CAD build for the part. Positions are in the model's coordinates, mm. A direction names the side the tool comes from. Give positions to 0.01 mm unless a question says otherwise; leave off trailing zeros. Loops run counter-clockwise (first coordinate to the right, second up) from the corner with the lowest first, then second, coordinate; pieces in that order, holes last.
```python
from build123d import *

# Parameters (mm, degrees)
SKETCH2_W                      = 230
SKETCH2_H                      = 283.251
BOSS_EXTRUDE1_DEPTH            = 10
SKETCH3_W                      = 10
SKETCH3_H                      = 283.251
BOSS_EXTRUDE2_DEPTH            = 170
M6_CLEARANCE_HOLE1_D           = 7
CUT_EXTRUDE1_DEPTH             = 327.431895271
CUT_EXTRUDE1_DEPTH_BACK        = 327.431895271
SKETCH7_R                      = 3.81
SKETCH7_R_2                    = 1.89865
SKETCH8_W                      = 6.35
SKETCH8_H                      = 38.1
CUT_EXTRUDE2_DEPTH             = 36.025
CUT_EXTRUDE3_DEPTH             = 6.35
CUT_EXTRUDE4_REACH             = 331.125
SKETCH11_R                     = 3.81
F_6_CLEARANCE_HOLE1_D          = 3.7973
F_6_CLEARANCE_HOLE1_DEPTH      = 3.65
CIRPATTERN1_COUNT              = 2
ENL_V_MAT_EXTRU_1_REACH        = 249.554
ESQUISSE1_R                    = 3.175
CBORE_FOR_M5_SHCS1_D           = 5.5
CBORE_FOR_M5_SHCS1_CBORE_D     = 10
CBORE_FOR_M5_SHCS1_CBORE_DEPTH = 5
CUT_EXTRUDE5_DEPTH             = 248.553594703
CUT_EXTRUDE5_DEPTH_BACK        = 248.553594703
SKETCH15_W                     = 58.825
SKETCH15_H                     = 59.331356017
CUT_EXTRUDE7_DEPTH             = 248.553594703
CUT_EXTRUDE7_DEPTH_BACK        = 248.553594703
SKETCH20_W                     = 0.765
SKETCH20_H                     = 59.331356017
FILLET2_R                      = 4
FILLET3_R                      = 144
FILLET4_R                      = 4
CUT_EXTRUDE8_REACH             = 335.853
CUT_EXTRUDE9_REACH             = 335.853
FILLET5_R                      = 8
FILLET6_R                      = 8
FILLET7_R                      = 10


with BuildPart() as part:
    # Sketch2 → Boss-Extrude1 (new body)
    with BuildSketch(Plane(origin=(0, 0, 0), x_dir=(1, 0, 0), z_dir=(0, 1, 0))):
        Rectangle(SKETCH2_W, SKETCH2_H)
    extrude(amount=BOSS_EXTRUDE1_DEPTH)

    # Sketch3 → Boss-Extrude2 (add)
    with BuildSketch(Plane(origin=(0, 0, 0), x_dir=(1, 0, 0), z_dir=(0, 1, 0))):
        with Locations((-120, 0)):
            Rectangle(SKETCH3_W, SKETCH3_H)
        with Locations((120, 0)):
            Rectangle(SKETCH3_W, SKETCH3_H)
    extrude(amount=BOSS_EXTRUDE2_DEPTH)

    # M6 Clearance Hole1 (through all)
    with Locations(Plane(origin=(0, 10, 0), x_dir=(1, 0, 0), z_dir=(0, 1, 0))):
        with Locations((-25, 25), (25, 25), (25, -25), (-25, -25)):
            Hole(M6_CLEARANCE_HOLE1_D / 2)

    # Sketch7 → Cut-Extrude1 (cut, two sides: drawn at the far end of the back side and taken through both)
    with BuildSketch(Plane.ZY.offset(-115).offset(-CUT_EXTRUDE1_DEPTH_BACK)):
        with Locations((0, 153.49)):
            Circle(SKETCH7_R)
        with Locations((0, 163.269)):
            Circle(SKETCH7_R_2)
        with Locations((6.914797213, 160.404797213)):
            Circle(SKETCH7_R_2)
        with Locations((9.779, 153.49)):
            Circle(SKETCH7_R_2)
        with Locations((6.914797213, 146.575202787)):
            Circle(SKETCH7_R_2)
        with Locations((0, 143.711)):
            Circle(SKETCH7_R_2)
        with Locations((-6.914797213, 146.575202787)):
            Circle(SKETCH7_R_2)
        with Locations((-9.779, 153.49)):
            Circle(SKETCH7_R_2)
        with Locations((-6.914797213, 160.404797213)):
            Circle(SKETCH7_R_2)
    extrude(amount=CUT_EXTRUDE1_DEPTH + CUT_EXTRUDE1_DEPTH_BACK, mode=Mode.SUBTRACT)

    # Sketch8 → Cut-Extrude2 (cut)
    with BuildSketch(Plane(origin=(0, 170, 0), x_dir=(1, 0, 0), z_dir=(0, 1, 0))):
        with Locations((121.825, 0)):
            Rectangle(SKETCH8_W, SKETCH8_H)
        with Locations((-121.825, 0)):
            Rectangle(SKETCH8_W, SKETCH8_H)
    extrude(amount=-CUT_EXTRUDE2_DEPTH, mode=Mode.SUBTRACT)

    # Sketch9 → Cut-Extrude3 (cut)
    with BuildSketch(Plane(origin=(125, 0, 0), x_dir=(0, 0, -1), z_dir=(1, 0, 0))):
        Polygon((72.294143983, 74.514), (72.294143983, 35.986), (34.274143983, 35.986), (34.274143983, 74.514), (34.274143983, 170), (72.294143983, 170), align=None)
    cut_extrude3 = extrude(amount=-CUT_EXTRUDE3_DEPTH, mode=Mode.SUBTRACT)

    # Sketch11 → Cut-Extrude4 (cut, up to next)
    with BuildSketch(Plane(origin=(118.65, 0, 0), x_dir=(0, 0, -1), z_dir=(1, 0, 0)), mode=Mode.PRIVATE) as cut_extrude4_sk1:
        with Locations((53.284143983, 55.25)):
            Circle(SKETCH11_R)
    cut_extrude4_tool1 = extrude(cut_extrude4_sk1.sketch, amount=-CUT_EXTRUDE4_REACH, mode=Mode.PRIVATE) & part.part
    cut_extrude4 = cut_extrude4_tool1.solids().sort_by_distance((118.65, 55.25, -53.284144))[0]
    add(cut_extrude4, mode=Mode.SUBTRACT)

    # #6 Clearance Hole1
    with Locations(Plane(origin=(118.65, 0, 0), x_dir=(0, 0, -1), z_dir=(1, 0, 0))):
        with Locations((53.284143983, 65.029), (43.505143983, 55.25), (63.063143983, 55.25), (53.284143983, 45.471)):
            f_6_clearance_hole1 = Hole(F_6_CLEARANCE_HOLE1_D / 2, depth=F_6_CLEARANCE_HOLE1_DEPTH)

    # CirPattern1: Cut-Extrude3, Cut-Extrude4, #6 Clearance Hole1 ×2 about axis
    cirpattern1_axis = Axis((0, 0, 0), (0, 1, 0))
    add([cut_extrude3.rotate(cirpattern1_axis, i * 360 / CIRPATTERN1_COUNT) for i in range(1, CIRPATTERN1_COUNT)], mode=Mode.SUBTRACT)
    add([cut_extrude4.rotate(cirpattern1_axis, i * 360 / CIRPATTERN1_COUNT) for i in range(1, CIRPATTERN1_COUNT)], mode=Mode.SUBTRACT)
    add([f_6_clearance_hole1.rotate(cirpattern1_axis, i * 360 / CIRPATTERN1_COUNT) for i in range(1, CIRPATTERN1_COUNT)], mode=Mode.SUBTRACT)

    # Esquisse1 → Enlèv. mat.-Extru.1 (cut, up to next)
    with BuildSketch(Plane(origin=(0, 10, 0), x_dir=(1, 0, 0), z_dir=(0, 1, 0)), mode=Mode.PRIVATE) as enl_v_mat_extru_1_sk1:
        with Locations(Location((53, 82.268595163, 0), (0, 0, 270))):
            Circle(ESQUISSE1_R)
    enl_v_mat_extru_1_tool1 = extrude(enl_v_mat_extru_1_sk1.sketch, amount=-ENL_V_MAT_EXTRU_1_REACH, mode=Mode.PRIVATE) & part.part
    # Esquisse1 → Enlèv. mat.-Extru.1 (cut, up to next)
    with BuildSketch(Plane(origin=(0, 10, 0), x_dir=(1, 0, 0), z_dir=(0, 1, 0)), mode=Mode.PRIVATE) as enl_v_mat_extru_1_sk2:
        with Locations(Location((53, -18.267555417, 0), (0, 0, 270))):
            Circle(ESQUISSE1_R)
    enl_v_mat_extru_1_tool2 = extrude(enl_v_mat_extru_1_sk2.sketch, amount=-ENL_V_MAT_EXTRU_1_REACH, mode=Mode.PRIVATE) & part.part
    add(enl_v_mat_extru_1_tool1.solids().sort_by_distance((53, 10, -82.268595))[0], mode=Mode.SUBTRACT)
    add(enl_v_mat_extru_1_tool2.solids().sort_by_distance((53, 10, 18.267555))[0], mode=Mode.SUBTRACT)

    # CBORE for M5 SHCS1 (through all)
    with Locations(Plane(origin=(0, 0, 0), x_dir=(-1, 0, 0), z_dir=(0, -1, 0))):
        with Locations((53, -24.299692803), (53, -124.835843383)):
            CounterBoreHole(CBORE_FOR_M5_SHCS1_D / 2, CBORE_FOR_M5_SHCS1_CBORE_D / 2, CBORE_FOR_M5_SHCS1_CBORE_DEPTH)

    # Sketch15 → Cut-Extrude5 (cut, two sides: drawn at the far end of the back side and taken through both)
    with BuildSketch(Plane(origin=(0, 10, 0), x_dir=(1, 0, 0), z_dir=(0, 1, 0)).offset(-CUT_EXTRUDE5_DEPTH_BACK)):
        with BuildLine():
            Line((125, 141.6255), (-125, 141.6255))
            Line((-125, 141.6255), (-125, 29.05))
            Line((-125, 29.05), (-64.845300659, 29.05))
            ThreePointArc((-64.845300659, 29.05), (-19.453683623, 68.340103242), (39.825, 58.845432215))
            Line((39.825, 58.845432215), (39.825, 95.443595163))
            Line((39.825, 95.443595163), (66.175, 95.443595163))
            Line((66.175, 95.443595163), (66.175, 82.294143983))
            Line((66.175, 82.294143983), (125, 82.294143983))
            Line((125, 82.294143983), (125, 141.6255))
        make_face()
        with BuildLine():
            Line((125, -141.6255), (125, -29.05))
            Line((125, -29.05), (64.845300659, -29.05))
            ThreePointArc((64.845300659, -29.05), (19.453683623, -68.340103242), (-39.825, -58.845432215))
            Line((-39.825, -58.845432215), (-39.825, -141.6255))
            Line((-39.825, -141.6255), (125, -141.6255))
        make_face()
        with Locations((-95.5875, -111.959821992)):
            Rectangle(SKETCH15_W, SKETCH15_H)
    extrude(amount=CUT_EXTRUDE5_DEPTH + CUT_EXTRUDE5_DEPTH_BACK, mode=Mode.SUBTRACT)

    # Sketch20 → Cut-Extrude7 (cut, two sides: drawn at the far end of the back side and taken through both)
    with BuildSketch(Plane(origin=(0, 10, 0), x_dir=(1, 0, 0), z_dir=(0, 1, 0)).offset(-CUT_EXTRUDE7_DEPTH_BACK)):
        with Locations((-65.7925, -111.959821992)):
            Rectangle(SKETCH20_W, SKETCH20_H)
        with BuildLine():
            Line((-39.824999998, -141.6255), (-39.824999998, -79.27802459))
            ThreePointArc((-39.824999998, -79.27802459), (-41.410278354, -80.751625782), (-41.995854347, -82.835302509))
            Line((-41.995854347, -82.835302509), (-41.995854347, -141.6255))
            Line((-41.995854347, -141.6255), (-39.824999998, -141.6255))
        make_face()
        with BuildLine():
            Line((39.825, 95.443595163), (66.175, 95.443595163))
            Line((66.175, 95.443595163), (66.175, 82.294143983))
            Line((66.175, 82.294143983), (65.41, 82.294143983))
            Line((65.41, 82.294143983), (65.41, 88.113136011))
            ThreePointArc((65.41, 88.113136011), (64.238427125, 90.941563136), (61.41, 92.113136011))
            Line((61.41, 92.113136011), (46, 92.113136011))
            ThreePointArc((46, 92.113136011), (43.171572875, 90.941563136), (42, 88.113136011))
            Line((42, 88.113136011), (42, 76.113136011))
            ThreePointArc((42, 76.113136011), (41.413209633, 74.02747065), (39.825, 72.553729459))
            Line((39.825, 72.553729459), (39.825, 95.443595163))
        make_face()
    extrude(amount=CUT_EXTRUDE7_DEPTH + CUT_EXTRUDE7_DEPTH_BACK, mode=Mode.SUBTRACT)

    # Fillet2
    fillet2_edges = [part.edges().sort_by_distance(p)[0] for p in [
        (-65.41, 5, 141.6255),
        (-41.995854347, 5, 141.6255),
    ]]
    fillet(fillet2_edges, radius=FILLET2_R)

    # Fillet3
    # the kernel refuses this fillet: 144 mm, written as the material it adds along each edge
    with BuildSketch(Plane(origin=(39.825, 0, -58.845432215), x_dir=(-0.9448497264443181, 0, -0.3275041899550252), z_dir=(0, 1, 0))) as fillet3_piece_1:
        with BuildLine():
            CenterArc((73.914316816, -139.111696925), FILLET3_R, 104.971721204, 13.852011514)
            Line((4.489524785, -12.952280901), (0, 0))
            ThreePointArc((0, 0), (18.356514745, -2.412072644), (36.713029491, 0))
        make_face()
    extrude(amount=10)
    with BuildSketch(Plane(origin=(-39.825, 10, 58.845432215), x_dir=(1.16727742405119e-10, 0, 1.0), z_dir=(0, -1, 0))) as fillet3_piece_2:
        with BuildLine():
            CenterArc((156.036482988, -48.451881806), FILLET3_R, 160.337962033, 17.363014277)
            ThreePointArc((12.15239164, -42.675355439), (9.492802158, -20.364752295), (0, 0))
            Line((0, 0), (20.432592375, 0))
        make_face()
    extrude(amount=10)

    # Fillet4
    fillet4_edges = [part.edges().sort_by_distance(p)[0] for p in [
        (-64.845300659, 5, -29.05),
        (64.845300659, 5, 29.05),
        (-65.41, 5, 82.294143983),
        (65.41, 5, -82.294143983),
    ]]
    fillet(fillet4_edges, radius=FILLET4_R)

    # Sketch22 → Cut-Extrude8 (cut, up to next)
    with BuildSketch(Plane.ZY.offset(125), mode=Mode.PRIVATE) as cut_extrude8_sk1:
        Polygon((26.622071991, 170), (82.294143983, 82.011), (82.294143983, 170), align=None)
    cut_extrude8_tool1 = extrude(cut_extrude8_sk1.sketch, amount=-CUT_EXTRUDE8_REACH, mode=Mode.PRIVATE) & part.part
    add(cut_extrude8_tool1.solids().sort_by_distance((-125, 140.670333, 63.736787))[0], mode=Mode.SUBTRACT)

    # Sketch23 → Cut-Extrude9 (cut, up to next)
    with BuildSketch(Plane(origin=(125, 0, 0), x_dir=(0, 0, -1), z_dir=(1, 0, 0)), mode=Mode.PRIVATE) as cut_extrude9_sk1:
        Polygon((29.05, 170), (82.294143983, 82.011), (82.294143983, 170), align=None)
    cut_extrude9_tool1 = extrude(cut_extrude9_sk1.sketch, amount=-CUT_EXTRUDE9_REACH, mode=Mode.PRIVATE) & part.part
    add(cut_extrude9_tool1.solids().sort_by_distance((125, 140.670333, -64.546096))[0], mode=Mode.SUBTRACT)

    # Fillet5
    fillet5_edges = [part.edges().sort_by_distance(p)[0] for p in [
        (-120, 170, -29.05),
        (120, 170, 29.05),
        (-120, 82.011, 82.294143983),
        (-120, 170, 26.622071991),
        (120, 170, -29.05),
        (120, 82.011, -82.294143983),
    ]]
    fillet(fillet5_edges, radius=FILLET5_R)

    # Fillet6
    fillet6_edges = [part.edges().sort_by_distance(p)[0] for p in [
        (-121.825, 157.905997776, 34.274143983),
    ]]
    fillet(fillet6_edges, radius=FILLET6_R)

    # Fillet7
    fillet7_edges = [part.edges().sort_by_distance(p)[0] for p in [
        (115, 10, -26.622071991),
        (-115, 10, 26.622071991),
    ]]
    fillet(fillet7_edges, radius=FILLET7_R)


solid = part.part
```
1. Saw through at B-B, the plane x = 53. List the corners of the cut face in (y, z), and give its area (3 significant figures).
Responses:
outline: (0, -92.11) - (10, -92.11) - (10, -85.44) - (0, -85.44) - close; (0, -79.09) - (10, -79.09) - (10, 15.09) - (0, 15.09) - close; (0, 21.44) - (10, 21.44) - (10, 47.33) - (0, 47.33) - close
area: 1,270 mm2
2. Pull direction Z, two halves, no side cores. Call faces 1 (the face through (-122, 97, 34.274)), 2 (the face through (125, 65, -13)), 3 (the face through (117.85, 125.61, -55.91)): released by +Z, released by -Z, zero draft, split by the parting line, or undercut.
Responses:
face 1: undercut
face 2: zero draft
face 3: released by -Z
3. Drop flat-ended pins along their axis: pin 1 (8 mm diameter, centred on y = 60.5, z = 50.5, fed in from +X); pin 2 (10 mm diameter, centred on y = 139.5, z = -40, fed in from +X); pin 3 (5 mm diameter, centred on y = 143.711, z = 0, fed in from -X); pin 4 (4 mm diameter, centred on x = 48, z = 30, fed in from -Y). Give the stop position or say it passes through.
Responses:
pin 1: stops at x = -115
pin 2: stops at x = 118.65
pin 3: stops at x = -118.65
pin 4: stops at y = 0
4. Tool access for faces 4 (the face through (-122, 66, 72.294)), 5 (the face through (115, 94, -26)), 6 (the face through (-65.41, 5, 112)): list every direction of +Z, -Z, +X, -X, +Y, -Y with a clear straight run to the whole face (end or side of a thin tool).
Responses:
face 4: -X, +Y
face 5: +Z, -Z, +Y
face 6: +Z, -X, +Y, -Y
5. Probe line 1 along X through (y, z) = (43.5, -3); line 2 along Y through (x, z) = (100, -14.5); line 3 along Z through (x, y) = (-116, 153). List the from-to ranges inside material, lowest first.
Responses:
line 1: x = -125 to -115, 115 to 125
line 2: y = 0 to 10
line 3: z = -29.05 to -11.61, -7.94 to -3.78, 3.78 to 7.94, 11.61 to 37.38
6. Saw through at D-D, the plane x = 25. List the corners of the cut face in (y, z).
Responses:
outline: (0, -70.8) - (10, -70.8) - (10, -28.5) - (0, -28.5) - close; (0, -21.5) - (10, -21.5) - (10, 21.5) - (0, 21.5) - close; (0, 28.5) - (10, 28.5) - (10, 66.51) - (0, 66.51) - close
7. Saw through at A-A, the plane y = 26. List the corners of the cut face in (x, z).
Responses:
outline: (-125, -29.05) - (-115, -29.05) - (-115, 82.29) - (-125, 82.29) - close; (115, -82.29) - (125, -82.29) - (125, 29.05) - (115, 29.05) - close
8. Saw through at C-C, the plane y = 120.5. List the corners of the cut face in (x, z).
Responses:
outline: (-125, -29.05) - (-115, -29.05) - (-115, 57.94) - (-118.65, 57.94) - (-118.65, 34.27) - (-125, 34.27) - close; (115, -59) - (118.65, -59) - (118.65, -34.27) - (125, -34.27) - (125, 29.05) - (115, 29.05) - close
